The model under review builds one solid part; all positions refer to its coordinate system, in mm. Give positions to 0.01 mm unless a question says otherwise; leave off trailing zeros. Order: outer loops, then holes, each group sorted by start corner. A loop starts at its lowest first (then second) coordinate and runs counter-clockwise, first axis right, second up. Notation, with made-up numbers: (48.25, 68.25) - (66.25, 68.25) arc R22 cw to (66.25, 83.25) - close; hole circle Ø6 at (29, 19.25). An arc over 180 degrees is marked (long way). Use CSV: the item, a comma, the result in double quotes.
```python
from build123d import *

# Parameters (mm, degrees)
REVOLVE2_ANGLE      = 180
SKETCH2_R           = 12.7
BOSS_EXTRUDE1_DEPTH = 2.54
REVOLVE3_ANGLE      = 180


with BuildPart() as part:
    # Sketch1 → Revolve2 (revolve)
    with BuildSketch(Plane(origin=(0, 0, 0), x_dir=(1, 0, 0), z_dir=(0, 1, 0))):
        with BuildLine():
            Line((0, -12.7), (0, 12.7))
            ThreePointArc((0, 12.7), (12.7, 0), (0, -12.7))
        make_face()
    revolve(axis=Axis((0, 0, 12.7), (0, 0, -1)), revolution_arc=REVOLVE2_ANGLE)

    # Sketch2 → Boss-Extrude1 (add)
    with BuildSketch(Plane(origin=(0, 0, 0), x_dir=(1, 0, 0), z_dir=(0, 1, 0))):
        with Locations(Location((0, 0, 0), (0, 0, 180))):
            Circle(SKETCH2_R)
    extrude(amount=BOSS_EXTRUDE1_DEPTH)

    # Sketch3 → Revolve3 (revolve)
    with BuildSketch(Plane(origin=(0, 2.54, 0), x_dir=(1, 0, 0), z_dir=(0, 1, 0))):
        with BuildLine():
            Line((0, 12.7), (0, -12.7))
            ThreePointArc((0, -12.7), (12.7, 0), (0, 12.7))
        make_face()
    revolve(axis=Axis((0, 2.54, -12.7), (0, 0, 1)), revolution_arc=REVOLVE3_ANGLE)


solid = part.part
```
Item 1: Clearance check with flat-ended pins moving along their axes: pin 1 (2 mm diameter, centred on y = -1, z = 3.5, fed in from -X); pin 2 (4 mm diameter, centred on x = -8.5, z = 7.5, fed in from +Y); pin 3 (6 mm diameter, centred on y = 2, z = -5, fed in from -X). State where each tip first meets the part, or that it passes through.
Results list:
pin 1,"stops at x = -12.42"
pin 2,"stops at y = 11.15"
pin 3,"stops at x = -12.54"
Item 2: Take a section at A-A, the plane z = 0. Give the boundary of the cut face in (x, y), and give its area (3 significant figures).
Results list:
outline,"(-12.7, 0) arc R12.7 ccw to (12.7, 0) - (12.7, 2.54) arc R12.7 ccw to (-12.7, 2.54) - close"
area,"571 mm2"
Item 3: Take a section at B-B, the plane x = 0. Give the boundary of the cut face in (y, z).
Results list:
outline,"(0, -12.7) - (2.54, -12.7) arc R12.7 ccw to (2.54, 12.7) - (0, 12.7) arc R12.7 ccw to start"
Item 4: Wall thickness on L1, parallel to Y at x = 0.25, z = -1; L2, parallel to Z at x = 6.5, y = -5.75; L3, parallel to Z at x = 11, y = -0.25: over which ranges is each line inside the solid? List them lowest first.
Results list:
L1,"y = -12.66 to 15.2"
L2,"z = -9.27 to 9.27"
L3,"z = -6.34 to 6.34"
Item 5: Take a section at C-C, the plane y = 5.75. Give the boundary of the cut face in (x, z).
Results list:
outline,"circle Ø24.58 at (0, 0)"
Item 6: Take a section at D-D, the plane y = 13.25. Give the boundary of the cut face in (x, z).
Results list:
outline,"circle Ø13.65 at (0, 0)"
